Input: part model. Units: mm. Frame: model coordinates. A direction names the side the tool comes from. Round coordinates to 2 decimals unless told otherwise and drop trailing zeros. Loops run counter-clockwise (first coordinate to the right, second up) from the corner with the lowest first, then second, coordinate; pieces in that order, holes last.
1) Section A-A, the plane z = -4. Return loops of the section in (x, y) (3 decimals).
2) Draft query along X for faces 1 (the face through (34.905, 9.392, -7.229)), 2 (the face through (-12.256, 13.808, -4.336)), 3 (the face through (0, 9, 0)). Return one class per face: pulls with the +X half, pulls with the -X half, needs draft (parallel to the pull), parting line crosses it, or undercut.
3) Section B-B, the plane y = 2.75. Return loops of the section in (x, z), and give its area (3 significant figures).
4) Access query for faces 4 (the face through (-8.977, 7.058, -1.545)), 5 (the face through (-25.536, 9.658, -6.084)), 6 (the face through (12, 8, -3.048)). Directions: +Z, -Z, +X, -X, +Y, -Y. A direction counts if a zero-diameter tool reaches every point of the face in a straight line with its end or side. Return the directions, or none.
5) Ray query, line 1 along X through (y, z) = (7.25, -5.5); line 2 along X through (y, z) = (10, -7.25); line 3 along X through (y, z) = (8.25, -5.25). Return the intervals inside material, ascending.
6) Section C-C, the plane x = -1. Return loops of the section in (y, z).
7) First-contact query: pin 1 (2 mm diameter, centred on x = 2, y = 14, fed in from -Z); pin 2 (3 mm diameter, centred on x = -9.525, y = 9.525, fed in from -Z); pin 3 (2 mm diameter, centred on x = -2, z = -6, fed in from -Y); pin 4 (6 mm diameter, centred on x = 9.525, y = 9.525, fed in from -Z). Flat tips, straight axial feed; report the tip coordinate or a pass-through.
from build123d import *

# Parameters (mm, degrees)
SKETCH1_R                      = 3.556
BOSS_EXTRUDE1_DEPTH            = 19.05
FILLET2_R                      = 2.54
F_8_0_199_DIAMETER_HOLE1_D     = 5.0546
F_8_0_199_DIAMETER_HOLE1_DEPTH = 9.149444958
F_8_0_199_DIAMETER_HOLE1_TIP   = 1.518555042
SKETCH11_R                     = 5.08
CUT_EXTRUDE1_DEPTH             = 2.54


with BuildPart() as part:
    # Sketch1 → Boss-Extrude1 (new body)
    with BuildSketch(Plane(origin=(0, 0, 0), x_dir=(1, 0, 0), z_dir=(0, 1, 0))):
        with BuildLine():
            Line((-31.75, 0), (31.75, 0))
            ThreePointArc((31.75, 0), (35.701312693, 9.539312693), (26.162, 5.588))
            Line((26.162, 5.588), (-26.162, 5.588))
            ThreePointArc((-26.162, 5.588), (-35.701312693, 9.539312693), (-31.75, 0))
        make_face()
        with Locations(Location((31.75, 5.588, 0), (0, 0, 90))):
            Circle(SKETCH1_R, mode=Mode.SUBTRACT)
        with Locations(Location((-31.75, 5.588, 0), (0, 0, 90))):
            Circle(SKETCH1_R, mode=Mode.SUBTRACT)
    extrude(amount=BOSS_EXTRUDE1_DEPTH)

    # Fillet2
    fillet2_edges = [part.edges().sort_by_distance(p)[0] for p in [
        (-26.162, 9.525, -5.588),
        (26.162, 9.525, -5.588),
    ]]
    fillet(fillet2_edges, radius=FILLET2_R)

    # #8 (0.199) Diameter Hole1
    with Locations(Plane.XY):
        with Locations((-9.525, 9.525), (9.525, 9.525)):
            Hole(F_8_0_199_DIAMETER_HOLE1_D / 2, depth=F_8_0_199_DIAMETER_HOLE1_DEPTH)
            with Locations((0, 0, -(F_8_0_199_DIAMETER_HOLE1_DEPTH + F_8_0_199_DIAMETER_HOLE1_TIP / 2))):  # 118° drill point
                Cone(0, F_8_0_199_DIAMETER_HOLE1_D / 2, F_8_0_199_DIAMETER_HOLE1_TIP, mode=Mode.SUBTRACT)

    # Sketch11 → Cut-Extrude1 (cut)
    with BuildSketch(Plane(origin=(0, 0, -5.588), x_dir=(-1, 0, 0), z_dir=(0, 0, -1))):
        with Locations((-9.525, 9.525)):
            Circle(SKETCH11_R)
        with Locations((9.525, 9.525)):
            Circle(SKETCH11_R)
    extrude(amount=-CUT_EXTRUDE1_DEPTH, mode=Mode.SUBTRACT)


solid = part.part
Final values:
1. outline: (-37.108, 0) - (-34.932, 0) - (-34.932, 19.05) - (-37.108, 19.05) - close; (-28.568, 0) - (28.568, 0) - (28.568, 19.05) - (-28.568, 19.05) - close; (34.932, 0) - (37.108, 0) - (37.108, 19.05) - (34.932, 19.05) - close; hole circle Ø10.16 at (-9.525, 9.525); hole circle Ø10.16 at (9.525, 9.525)
2. face 1: undercut
2. face 2: undercut
2. face 3: needs draft
3. outline: (-31.75, 0) arc R5.59 ccw (long way) to (-26.44, -7.33) arc R2.54 cw to (-24.03, -5.59) - (24.03, -5.59) arc R2.54 cw to (26.44, -7.33) arc R5.59 ccw (long way) to (31.75, 0) - close; hole circle Ø7.11 at (-31.75, -5.59); hole circle Ø7.11 at (31.75, -5.59)
3. area: 424 mm2
4. face 4: +Z, -Z
4. face 5: -Z, +Y, -Y
4. face 6: -Z
5. line 1: x = -37.34 to -35.3, -28.2 to -14.07, -4.98 to 4.98, 14.07 to 28.2, 35.3 to 37.34
5. line 2: x = -37.09 to -34.89, -28.61 to -26.41, 26.41 to 28.61, 34.89 to 37.09
5. line 3: x = -37.33 to -35.29, -28.21 to -14.44, -4.61 to 4.61, 14.44 to 28.21, 35.29 to 37.33
6. outline: (0, -5.59) - (19.05, -5.59) - (19.05, 0) - (0, 0) - close
7. pin 1: stops at z = -5.59
7. pin 2: passes through
7. pin 3: stops at y = 0
7. pin 4: stops at z = -3.05
